For this review, take the finished solid that the model builds, in its own axes (mm). Face numbers are marked on the shaded views. A direction names the side the tool comes from. Round coordinates to 2 decimals unless told otherwise and drop trailing zeros. Write each loop counter-clockwise with the first axis right and the second up, starting at its lowest first coordinate (ties: lowest second). Pieces come first, ordered by that corner, then holes. Notation, with made-up numbers: (62.25, 22) -> (82.25, 22) arc R24 ccw to (82.25, 54) -> close; hole circle Ø7 at (-11, 8.5). An arc over 180 degrees is marked (long way). Answer in a Markdown table with one row per item.
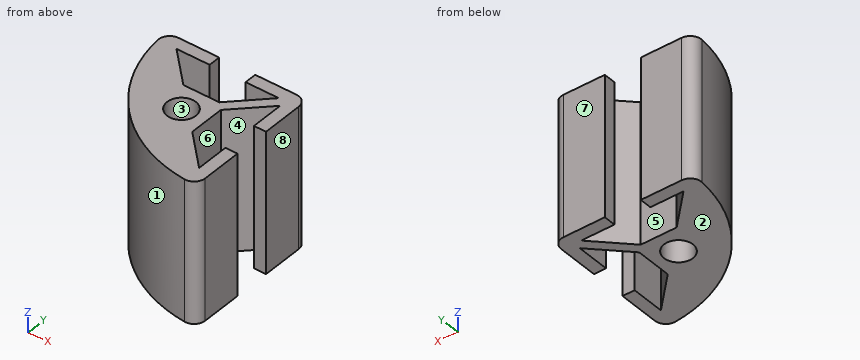
from build123d import *

# Parameters (mm, degrees)
SKETCH002_R     = 2.6035
PAD001_DEPTH    = 25.4
POCKET001_DEPTH = 25.401
FILLET001_R     = 2


with BuildPart() as part:
    # Sketch002 → Pad001 (new body)
    with BuildSketch(Plane.XY):
        with BuildLine():
            Line((12.7, -12.7), (12.7, 12.7))
            Line((12.7, 12.7), (-12.7, 12.7))
            ThreePointArc((-12.7, 12.7), (-5.260512, -5.260512), (12.7, -12.7))
        make_face()
        Circle(SKETCH002_R, mode=Mode.SUBTRACT)
    extrude(amount=PAD001_DEPTH)

    # Sketch003 (on Face6 of Pad001) → Pocket001 (cut, through all)
    with BuildSketch(Plane.XY.offset(25.4)):
        Polygon((-3.2512, 4.5212), (3.2512, 4.5212), (9.2456, 10.5156), (3.2512, 10.5156), (3.2512, 12.7), (-3.2512, 12.7), (-3.2512, 10.5156), (-9.2456, 10.5156), align=None)
        Polygon((4.5212, 3.2512), (4.5212, -3.2512), (10.5156, -9.2456), (10.5156, -3.2512), (12.7, -3.2512), (12.7, 3.2512), (10.5156, 3.2512), (10.5156, 9.2456), align=None)
    extrude(amount=-POCKET001_DEPTH, mode=Mode.SUBTRACT)

    # Fillet001
    fillet001_edges = [part.edges().sort_by_distance(p)[0] for p in [
        (12.7, 12.7, 12.7),
        (12.7, -12.7, 12.7),
        (-12.7, 12.7, 12.7),
    ]]
    fillet(fillet001_edges, radius=FILLET001_R)


solid = part.part
1) For the marked faces 4, 5, 6, 7 and 8, list the 3-axis set-ups (+Z, -Z, +X, -X, +Y, -Y) from which the entire face can be reached by the end or side of a thin tool; tool diameter is ignored.
Solved:
| item | result |
|---|---|
| face 4 | +Z, -Z |
| face 5 | +Z, -Z, +Y |
| face 6 | +Z, -Z, +X |
| face 7 | +Z, -Z, +X, -X, +Y |
| face 8 | +Z, -Z, +X, +Y, -Y |
2) Consider section D-D on x = 0. State the section outline as (y, z) points, then the cut area to 3 significant figures.
Solved:
| item | result |
|---|---|
| outline | (-9.3, 0) -> (-2.6, 0) -> (-2.6, 25.4) -> (-9.3, 25.4) -> close; (2.6, 0) -> (4.52, 0) -> (4.52, 25.4) -> (2.6, 25.4) -> close |
| area | 219 mm² |
3) For line 1 (X direction, y = 9, z = 22.5); line 2 (Y direction, x = 6.5, z = 15.5); line 3 (Y direction, x = 0, z = 6.25), list the stretches that pass through material, from the lowest coordinate up. Write a range as [from, to].
Solved:
| item | result |
|---|---|
| line 1 | [-12.43, -7.73], [7.73, 10.27], [10.52, 12.7] |
| line 2 | [-11.93, -5.23], [5.23, 7.77], [10.52, 12.7] |
| line 3 | [-9.3, -2.6], [2.6, 4.52] |
4) Mouldability with a two-part tool opening along X and no side actions: class the marked faces 1, 2 and 3 as pulls with the +X half, pulls with the -X half, needs draft (parallel to the pull), parting line crosses it, or undercut.
Solved:
| item | result |
|---|---|
| face 1 | pulls with the -X half |
| face 2 | needs draft |
| face 3 | undercut |
5) Consider section B-B on y = 1.25. State the section outline as (x, z) points.
Solved:
| item | result |
|---|---|
| outline | (-9.97, 0) -> (-2.28, 0) -> (-2.28, 25.4) -> (-9.97, 25.4) -> close; (2.28, 0) -> (4.52, 0) -> (4.52, 25.4) -> (2.28, 25.4) -> close |
6) Consider section C-C on x = 6.5. State the section outline as (y, z) points, then the cut area to 3 significant figures.
Solved:
| item | result |
|---|---|
| outline | (-11.93, 0) -> (-5.23, 0) -> (-5.23, 25.4) -> (-11.93, 25.4) -> close; (5.23, 0) -> (7.77, 0) -> (7.77, 25.4) -> (5.23, 25.4) -> close; (10.52, 0) -> (12.7, 0) -> (12.7, 25.4) -> (10.52, 25.4) -> close |
| area | 290 mm² |
7) Consider section A-A on z = 4.5. State the section outline as (x, y) points.
Solved:
| item | result |
|---|---|
| outline | (-12.61, 10.53) arc R25.4 ccw to (10.53, -12.61) arc R2 ccw to (12.7, -10.61) -> (12.7, -3.25) -> (10.52, -3.25) -> (10.52, -9.25) -> (4.52, -3.25) -> (4.52, 3.25) -> (10.52, 9.25) -> (10.52, 3.25) -> (12.7, 3.25) -> (12.7, 10.7) arc R2 ccw to (10.7, 12.7) -> (3.25, 12.7) -> (3.25, 10.52) -> (9.25, 10.52) -> (3.25, 4.52) -> (-3.25, 4.52) -> (-9.25, 10.52) -> (-3.25, 10.52) -> (-3.25, 12.7) -> (-10.61, 12.7) arc R2 ccw to start; hole circle Ø5.21 at (0, 0) |
8) Clearance check with flat-ended pins moving along their axes: pin 1 Ø5 at (x, z) = (0.5, 17.5) entering from +Y; pin 2 Ø3 at (y, z) = (-7.5, 15) entering from -X; pin 3 Ø2 at (y, z) = (1, 15.5) entering from +X; pin 4 Ø12 at (x, z) = (7.5, 9.5) entering from -Y. State where each tip first meets the part, or that it passes through.
Solved:
| item | result |
|---|---|
| pin 1 | y = 4.52 |
| pin 2 | x = -4.49 |
| pin 3 | x = 4.52 |
| pin 4 | y = -12.61 |
